```python
from build123d import *

# Parameters (mm, degrees)
SKETCH_1_W          = 100
SKETCH_1_H          = 100
SKETCH_1_R          = 1.6
F_100X100_1P6_DEPTH = 1.6
EXTRUDE_START       = -8
SKETCH_2_W          = 4
SKETCH_2_H          = 58
EXTRUDE_284_DEPTH   = 8
SKETCH_3_W          = 4
SKETCH_3_H          = 58
EXTRUDE_361_DEPTH   = 8
EXTRUDE_START_2     = -16
SKETCH_4_W          = 32
SKETCH_4_H          = 47
EXTRUDE_435_DEPTH   = 16
EXTRUDE_START_3     = -12
SKETCH_5_W          = 20
SKETCH_5_H          = 10
EXTRUDE_509_DEPTH   = 12
EXTRUDE_START_4     = -10
SKETCH_6_W          = 12
SKETCH_6_H          = 10
EXTRUDE_583_DEPTH   = 10
SKETCH_7_W          = 12
SKETCH_7_H          = 10
EXTRUDE_657_DEPTH   = 10


with BuildPart() as part:
    # 草图1 → 100x100_板厚1p6 (new body)
    with BuildSketch(Plane.XY):
        with Locations((50, 50)):
            Rectangle(SKETCH_1_W, SKETCH_1_H)
        with Locations((5, 5)):
            Circle(SKETCH_1_R, mode=Mode.SUBTRACT)
        with Locations((95, 5)):
            Circle(SKETCH_1_R, mode=Mode.SUBTRACT)
        with Locations((5, 95)):
            Circle(SKETCH_1_R, mode=Mode.SUBTRACT)
        with Locations((95, 95)):
            Circle(SKETCH_1_R, mode=Mode.SUBTRACT)
    extrude(amount=F_100X100_1P6_DEPTH)

    # 草图2 → Extrude 284 (add)
    with BuildSketch(Plane.XY.offset(EXTRUDE_START)):
        with Locations((28, 49)):
            Rectangle(SKETCH_2_W, SKETCH_2_H)
    extrude(amount=EXTRUDE_284_DEPTH)

    # 草图3 → Extrude 361 (add)
    with BuildSketch(Plane.XY.offset(EXTRUDE_START)):
        with Locations((72, 49)):
            Rectangle(SKETCH_3_W, SKETCH_3_H)
    extrude(amount=EXTRUDE_361_DEPTH)

    # 草图4 → Extrude 435 (add)
    with BuildSketch(Plane.XY.offset(EXTRUDE_START_2)):
        with Locations((50, 49.5)):
            Rectangle(SKETCH_4_W, SKETCH_4_H)
    extrude(amount=EXTRUDE_435_DEPTH)

    # 草图5 → Extrude 509 (add)
    with BuildSketch(Plane.XY.offset(EXTRUDE_START_3)):
        with Locations((50, 8)):
            Rectangle(SKETCH_5_W, SKETCH_5_H)
    extrude(amount=EXTRUDE_509_DEPTH)

    # 草图6 → Extrude 583 (add)
    with BuildSketch(Plane.XY.offset(EXTRUDE_START_4)):
        with Locations((40, 90)):
            Rectangle(SKETCH_6_W, SKETCH_6_H)
    extrude(amount=EXTRUDE_583_DEPTH)

    # 草图7 → Extrude 657 (add)
    with BuildSketch(Plane.XY.offset(EXTRUDE_START_4)):
        with Locations((60, 90)):
            Rectangle(SKETCH_7_W, SKETCH_7_H)
    extrude(amount=EXTRUDE_657_DEPTH)


solid = part.part
```
Could you check a few things on this model? Use its own coordinates, in mm. A direction names the side the tool comes from. Round coordinates to 2 decimals unless told otherwise and drop trailing zeros. Write each loop counter-clockwise with the first axis right and the second up, starting at its lowest first coordinate (ties: lowest second). Pieces come first, ordered by that corner, then holes. Notation, with made-up numbers: M 80,39 L 100,39 A19 cw 100,51 Z; hole C 86.25,-26.5 d6. An arc over 180 degrees is marked long. Write each question's results on one line, items separated by ' | '. Start each with the question number.
1. Thinking about a two-plate mould opening in X: for faces 5 (the face through (60, 8, -6)), 6 (the face through (26, 49, -4)), 7 (the face through (93.4, 95.07, 0.79)), 8 (the face through (30, 49, -4)), which applies, +X half, -X half, draft (parallel to the pull), parting line (faces both ways), or undercut?
2. Imagine slicing it at A-A on z = -6. List the corners of the cut face in (x, y) for me.
3. Imagine slicing it at C-C on y = 90. List the corners of the cut face in (x, z) for me.
4. I need wall thicknesses on L1, parallel to X at y = 29, z = -6.25; L2, parallel to Y at x = 5, z = 1.15; L3, parallel to Y at x = 58, z = -9.75. Which ranges of each line are inside material? Lowest first, please. Write a range as from..to.
5. Imagine slicing it at D-D on x = 50.5. List the corners of the cut face in (y, z) for me.
6. On a 3-axis mill with a long thin cutter (end or side, diameter ignored), from which of +Z, -Z, +X, -X, +Y, -Y can I reach the whole of each face in a straight line? I mean faces 1 (the face through (60, 90, -10)), 2 (the face through (70, 49, -4)), 3 (the face through (28, 20, -4)), 4 (the face through (60, 85, -5)). Say none if no direction works.
7. I'm going to push flat-ended pins straight in: pin 1 Ø1.5 at (x, y) = (81.5, 18.5) entering from -Z; pin 2 Ø5 at (y, z) = (55.5, -4.5) entering from -X; pin 3 Ø6 at (x, z) = (46.5, -3.5) entering from -Y. Where does each tip first touch, or does it pass through?
8. Imagine slicing it at B-B on x = 5. List the corners of the cut face in (y, z) for me.
Result sheet:
1) face 5: +X half | face 6: -X half | face 7: undercut | face 8: undercut
2) outline: M 26,20 L 30,20 L 30,78 L 26,78 Z; M 34,26 L 66,26 L 66,73 L 34,73 Z; M 34,85 L 46,85 L 46,95 L 34,95 Z; M 40,3 L 60,3 L 60,13 L 40,13 Z; M 54,85 L 66,85 L 66,95 L 54,95 Z; M 70,20 L 74,20 L 74,78 L 70,78 Z
3) outline: M 0,0 L 34,0 L 34,-10 L 46,-10 L 46,0 L 54,0 L 54,-10 L 66,-10 L 66,0 L 100,0 L 100,1.6 L 0,1.6 Z
4) L1: x = 26..30, 34..66, 70..74 | L2: y = 0..3.4, 6.6..93.4, 96.6..100 | L3: y = 3..13, 26..73, 85..95
5) outline: M 0,0 L 3,0 L 3,-12 L 13,-12 L 13,0 L 26,0 L 26,-16 L 73,-16 L 73,0 L 100,0 L 100,1.6 L 0,1.6 Z
6) face 1: -Z, +X, -X, +Y | face 2: -Z, +Y, -Y | face 3: -Z, +X, -X, -Y | face 4: -Z, +X, -X
7) pin 1: stops at z = 0 | pin 2: stops at x = 26 | pin 3: stops at y = 3
8) outline: M 0,0 L 3.4,0 L 3.4,1.6 L 0,1.6 Z; M 6.6,0 L 93.4,0 L 93.4,1.6 L 6.6,1.6 Z; M 96.6,0 L 100,0 L 100,1.6 L 96.6,1.6 Z
